Autodesk Inventor part; units mm, degrees
ref_plane "YZ Plane" through (0, 0, 0) normal (1, 0, 0) x (0, 1, 0)
ref_plane "XZ Plane" through (0, 0, 0) normal (0, 1, 0) x (-1, 0, 0)
sketch "Sketch1" plane through (0, 0, 0) normal (0, 1, 0) x (-1, 0, 0)
  line L0 (101.6, 12.7) -> (-101.6, 12.7)
  line L1 (-101.6, 12.7) -> (-101.6, -12.7)
  line L2 (-101.6, -12.7) -> (101.6, -12.7)
  line L3 (101.6, -12.7) -> (101.6, 12.7)
  line L4 (101.6, 12.7) -> (-101.6, -12.7) construction
  line L5 (-101.6, 12.7) -> (101.6, -12.7) construction
  point P0 (0, 0)
  dimension "d0" = 203.2
  dimension "d1" = 25.4
extrude "Extrusion1" add sketch "Sketch1" along normal mid plane 25.4
sketch "Sketch3" plane through (0, 12.7, 0) normal (0, 1, 0) x (1, 0, 0)
  line L0 (-101.6, -6.858) -> (38.1, -6.858)
  line L1 (38.1, -6.858) -> (38.1, 6.858)
  line L2 (38.1, 6.858) -> (-101.6, 6.858)
  line L3 (-101.6, 6.858) -> (-101.6, -6.858)
  line L4 (-101.6, -6.858) -> (38.1, 6.858) construction
  line L5 (38.1, -6.858) -> (-101.6, 6.858) construction
  line L6 (-101.6, 12.7) -> (-101.6, -12.7)
  point P0 (0, 0)
  point P1 (-31.75, 0)
  dimension "d7" = 0
  dimension "d8" = 13.716
  dimension "d9" = 139.7
extrude "Extrusion2" cut sketch "Sketch3" against normal through all
sketch "Sketch4" plane through (0, 12.7, 0) normal (0, 1, 0) x (1, 0, 0)
  line L0 (101.6, 12.7) -> (-101.6, 12.7)
  line L1 (101.6, 12.7) -> (63.5, 12.7)
  line L2 (63.5, 12.7) -> (63.5, 6.35)
  line L3 (63.5, 6.35) -> (101.6, 6.35)
  line L4 (101.6, 6.35) -> (101.6, 12.7)
  line L5 (101.6, 0) -> (38.1, 0) construction
  line L6 (38.1, 6.858) -> (38.1, -6.858) construction
  point P0 (0, 0)
  dimension "d12" = 38.1
  dimension "d13" = 6.35
extrude "Extrusion3" cut sketch "Sketch4" against normal through all
mirror "Mirror1" about plane through (0, 0, 0) normal (0, 0, 1) of "Extrusion3"
sketch "Sketch5" plane through (-101.6, -12.7, 12.7) normal (0, 0, 1) x (1, 0, 0)
  circle A0 centre (12.7, 12.7) radius 5.2705
  circle A1 centre (190.5, 12.7) radius 5.2705
  line L0 (0, 0) -> (0, 25.4)
  line L1 (203.2, 25.4) -> (203.2, 0)
  point P0 (101.6, 12.7)
  dimension "d16" = 10.541
  dimension "d17" = 12.7
  dimension "d18" = 12.7
extrude "Extrusion4" cut sketch "Sketch5" against normal through all
properties part number "connectingRodV02-4-in"
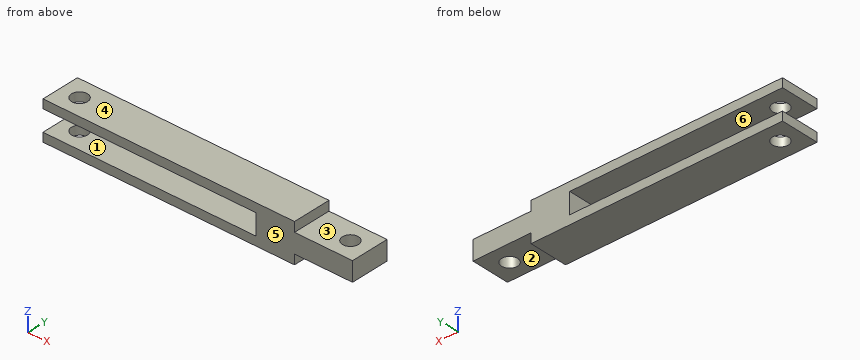
For this review, take the finished solid that the model builds, in its own axes (mm). Face numbers are marked on the shaded views. A direction names the side the tool comes from. Round coordinates to 2 decimals unless told otherwise and drop trailing zeros. Loops run counter-clockwise (first coordinate to the right, second up) from the corner with the lowest first, then second, coordinate; pieces in that order, holes last. Notation, with made-up numbers: (-37.75, 44.25) - (1.25, 44.25) arc R24 cw to (1.25, 57.25) - close; hole circle Ø11 at (-23, 60). An arc over 180 degrees is marked (long way). One line per item, written item: value. Start each with the question number.
Item 1: Take a section at D-D (y = 0). Give the boundary of the cut face in (x, z).
Item 2: Take a section at A-A (x = 88.9). Give the boundary of the cut face in (y, z).
Item 3: Clearance check with flat-ended pins moving along their axes: pin 1 Ø3 at (y, z) = (-5, 9.5) entering from +X; pin 2 Ø12.5 at (x, y) = (73.5, -1) entering from +Z; pin 3 Ø4 at (y, z) = (-3.5, -1) entering from -X. State where each tip first meets the part, or that it passes through.
Item 4: For L1, parallel to Y at x = -88.9, z = -11.1; L2, parallel to Z at x = -51, y = -6.5; L3, parallel to X at y = -10, z = -1.5, list the stretches that pass through material, from the lowest coordinate up.
Item 5: Take a section at B-B (x = -88.9). Give the boundary of the cut face in (y, z).
Item 6: Take a section at C-C (z = -10). Give the boundary of the cut face in (x, y).
Item 7: The part is to be moulded in two halves that separate along Z. For the marked faces 4, 5 and 6, say which applies: +Z half, -Z half, draft (parallel to the pull), parting line (faces both ways), or undercut.
Item 8: For the marked faces 1, 2 and 3, list the 3-axis set-ups (+Z, -Z, +X, -X, +Y, -Y) from which the entire face can be reached by the end or side of a thin tool; tool diameter is ignored.
Answer below:
1. outline: (-101.6, -12.7) - (-94.17, -12.7) - (-94.17, -6.86) - (-101.6, -6.86) - close; (-101.6, 6.86) - (-94.17, 6.86) - (-94.17, 12.7) - (-101.6, 12.7) - close; (-83.63, -12.7) - (63.5, -12.7) - (63.5, -6.35) - (83.63, -6.35) - (83.63, 6.35) - (63.5, 6.35) - (63.5, 12.7) - (-83.63, 12.7) - (-83.63, 6.86) - (38.1, 6.86) - (38.1, -6.86) - (-83.63, -6.86) - close; (94.17, -6.35) - (101.6, -6.35) - (101.6, 6.35) - (94.17, 6.35) - close
2. outline: (-12.7, -6.35) - (-5.27, -6.35) - (-5.27, 6.35) - (-12.7, 6.35) - close; (5.27, -6.35) - (12.7, -6.35) - (12.7, 6.35) - (5.27, 6.35) - close
3. pin 1: stops at x = 63.5
3. pin 2: stops at z = 6.35
3. pin 3: stops at x = 38.1
4. L1: y = -12.7 to -5.27, 5.27 to 12.7
4. L2: z = -12.7 to -6.86, 6.86 to 12.7
4. L3: x = 38.1 to 101.6
5. outline: (-12.7, -12.7) - (-5.27, -12.7) - (-5.27, -6.86) - (-12.7, -6.86) - close; (-12.7, 6.86) - (-5.27, 6.86) - (-5.27, 12.7) - (-12.7, 12.7) - close; (5.27, -12.7) - (12.7, -12.7) - (12.7, -6.86) - (5.27, -6.86) - close; (5.27, 6.86) - (12.7, 6.86) - (12.7, 12.7) - (5.27, 12.7) - close
6. outline: (-101.6, -12.7) - (63.5, -12.7) - (63.5, 12.7) - (-101.6, 12.7) - close; hole circle Ø10.54 at (-88.9, 0)
7. face 4: +Z half
7. face 5: draft
7. face 6: undercut
8. face 1: -X, +Y, -Y
8. face 2: -Z, +X, +Y, -Y
8. face 3: +Z, +X, +Y, -Y
